The model under review builds one solid part; all positions refer to its coordinate system, in mm. A direction names the side the tool comes from. Round coordinates to 2 decimals unless told otherwise and drop trailing zeros. Loops run counter-clockwise (first coordinate to the right, second up) from the corner with the lowest first, then second, coordinate; pieces in that order, holes last. Notation, with made-up numbers: (87, 22.5) - (104, 22.5) arc R16 cw to (104, 47.5) - close; hole circle Ø7 at (29.25, -1). An arc over 180 degrees is marked (long way). Answer as CSV lines item,"result".
Autodesk Inventor part; units mm, degrees
ref_plane "YZ Plane" through (0, 0, 0) normal (1, 0, 0) x (0, 1, 0)
ref_plane "XZ Plane" through (0, 0, 0) normal (0, 1, 0) x (-1, 0, 0)
ref_plane "XY Plane" through (0, 0, 0) normal (0, 0, 1) x (1, 0, 0)
sketch "Esquisse1" plane through (0, 0, 0) normal (0, 0, 1) x (1, 0, 0)
  line L0 (17.5, -109.2) -> (17.5, 0)
  line L1 (17.5, 0) -> (-17.5, 0)
  line L2 (-17.5, 0) -> (-17.5, -109.2)
  arc A0 (-17.5, -109.2) -> (17.5, -109.2) centre (0, -109.2) ccw
  arc A1 (-3.875, -116.7) -> (3.875, -116.7) centre (0, -116.7) ccw
  arc A2 (6.5, -101.7) -> (-6.5, -101.7) centre (0, -101.7) ccw
  line L3 (-3.875, -111.7) -> (-3.875, -116.7)
  line L4 (3.875, -116.7) -> (3.875, -111.7)
  line L5 (-6.5, -101.7) -> (-6.5, -104.7)
  line L6 (-6.5, -104.7) -> (-3.875, -111.7)
  line L7 (3.875, -111.7) -> (6.5, -104.7)
  line L8 (6.5, -104.7) -> (6.5, -101.7)
  point P0 (0, 0)
  point P1 (0, 0)
  dimension "d0" = 35
  dimension "d1" = 126.7
  dimension "d3" = 3
  dimension "d4" = 6.5
  dimension "d5" = 5
  dimension "d6" = 15
  dimension "d7" = 116.7
  dimension "d8" = 3.875
extrude "Embase" add sketch "Esquisse1" along normal blind 2
sketch "Esquisse2" plane through (0, 0, 2) normal (0, 0, 1) x (1, 0, 0)
  line L0 (-17.5, -15) -> (17.5, -15)
  line L1 (17.5, -15) -> (17.5, 0)
  line L2 (17.5, 0) -> (-17.5, 0)
  line L3 (-17.5, 0) -> (-17.5, -15)
  line L4 (17.5, 0) -> (-17.5, 0)
  line L5 (-17.5, 0) -> (-17.5, -109.2)
  line L6 (17.5, -109.2) -> (17.5, 0)
  point P0 (0, 0)
  dimension "d11" = 15
extrude "Support" add sketch "Esquisse2" along normal blind 20
sketch "Esquisse3" plane through (-17.5, -15, 2) normal (0, -1, 0) x (1, 0, 0)
  line L0 (0, -2) -> (0, 20)
  point P0 (17.5, -2)
  point P1 (10, 9)
  point P2 (25, 9)
  point P3 (0, 9)
  dimension "Entraxe" = 15
  dimension "d15" = 7.5
hole "Passage vis" at (-7.5, -15, 11) at (7.5, -15, 11) direction (0, 1, 0) diameter 5.5 end through all counterbore diameter 10 counterbore depth 5.5
fillet "Congé1" radius 4 3 edges at (-17.5, -7.5, 22) (17.5, -7.5, 22) (0, -15, 2)
fillet "Congé1" radius 5 4 edges at (3.875, -111.7, 1) (6.5, -104.7, 1) (-6.5, -104.7, 1) (-3.875, -111.7, 1)
fillet "Congé2" radius 1 15 edges at (16.3286, -15, 20.8286) (17.5, -15, 12) (17.5, -16.1714, 3.1714) (17.5, -64.0997, 2) (0, -126.7, 2) (-17.5, -64.0998, 2) (-17.5, -16.1714, 3.1714) (-17.5, -15, 12) (-16.3286, -15, 20.8286) (0, -15, 22) (-16.3286, 0, 20.8286) (-17.5, 0, 9.0003) (16.3286, 0, 20.8286) (17.5, 0, 9.0003) (0, 0, 22)
properties part number "Bras" material "Plastique ABS"
1. Clearance check with flat-ended pins moving along their axes: pin 1 (11 mm diameter, centred on x = -8, z = 12.5, fed in from -Y); pin 2 (5 mm diameter, centred on x = -8.5, z = 11, fed in from -Y); pin 3 (1 mm diameter, centred on y = -115, z = 0.5, fed in from -X). State where each tip first meets the part, or that it passes through.
Numbers:
pin 1,"stops at y = -15"
pin 2,"stops at y = -9.5"
pin 3,"stops at x = -16.68"
2. Draft analysis for pull direction X (two halves, no side actions). For faces 1 (the face through (0, -7, 22)), 2 (the face through (8.55, -4.68, 8.46)), 3 (the face through (0.385, -126.696, 0.493)), state which applies: +X half, -X half, draft (parallel to the pull), parting line (faces both ways), or undercut.
Numbers:
face 1,"draft"
face 2,"undercut"
face 3,"parting line"
3. Wall thickness on probe 1 along X at (y, z) = (-11.6, 11); probe 2 along X at (y, z) = (-3, 11); probe 3 along Z at (x, y) = (7, -11): over which ranges is each line inside the solid? List them lowest first.
Numbers:
probe 1,"x = -17.5 to -12.5, -2.5 to 2.5, 12.5 to 17.5"
probe 2,"x = -17.5 to -10.25, -4.75 to 4.75, 10.25 to 17.5"
probe 3,"z = 0 to 6.03, 15.97 to 22"
4. Tool access review of faces 4 (the face through (-0.1, -95.2, 1)), 5 (the face through (-16.297, -7.591, 20.859)), 6 (the face through (0, -72, 2)), 7 (the face through (-6.45, -4.68, 8.46)), 8 (the face through (-9, -12.21, 6.23)): name each direction out of +Z, -Z, +X, -X, +Y, -Y from which nothing blocks a thin tool from reaching the whole face with its end or side.
Numbers:
face 4,"+Z, -Z"
face 5,"+Z, -X, +Y, -Y"
face 6,"+Z, +X, -X, -Y"
face 7,"+Y, -Y"
face 8,"-Y"
5. Take a section at B-B (y = -34). State the section outline as (x, z) points.
Numbers:
outline,"(-17.5, 0) - (17.5, 0) - (17.5, 1) arc R1 ccw to (16.5, 2) - (-16.5, 2) arc R1 ccw to (-17.5, 1) - close"
6. Take a section at A-A (z = 11). State the section outline as (x, y) points, plus the area to 3 significant figures.
Numbers:
outline,"(-17.5, -14) arc R1 ccw to (-16.5, -15) - (-12.5, -15) - (-12.5, -9.5) - (-10.25, -9.5) - (-10.25, 0) - (-16.5, 0) arc R1 ccw to (-17.5, -1) - close; (-4.75, -9.5) - (-2.5, -9.5) - (-2.5, -15) - (2.5, -15) - (2.5, -9.5) - (4.75, -9.5) - (4.75, 0) - (-4.75, 0) - close; (10.25, -9.5) - (12.5, -9.5) - (12.5, -15) - (16.5, -15) arc R1 ccw to (17.5, -14) - (17.5, -1) arc R1 ccw to (16.5, 0) - (10.25, 0) - close"
area,"310 mm²"
